Part print with two shaded views. Sizes in mm from the minimum x, y, z corner. Round coordinates to 2 decimals unless told otherwise and drop trailing zeros. Order: outer loops, then holes, each group sorted by start corner. A loop starts at its lowest first (then second) coordinate and runs counter-clockwise, first axis right, second up. Notation, with made-up numbers: M 52,-11 L 82,-11 A19 cw 82,22 Z; hole C 18,-36 d5. An arc over 180 degrees is marked long. Answer as a JSON object with one key per item and string values.
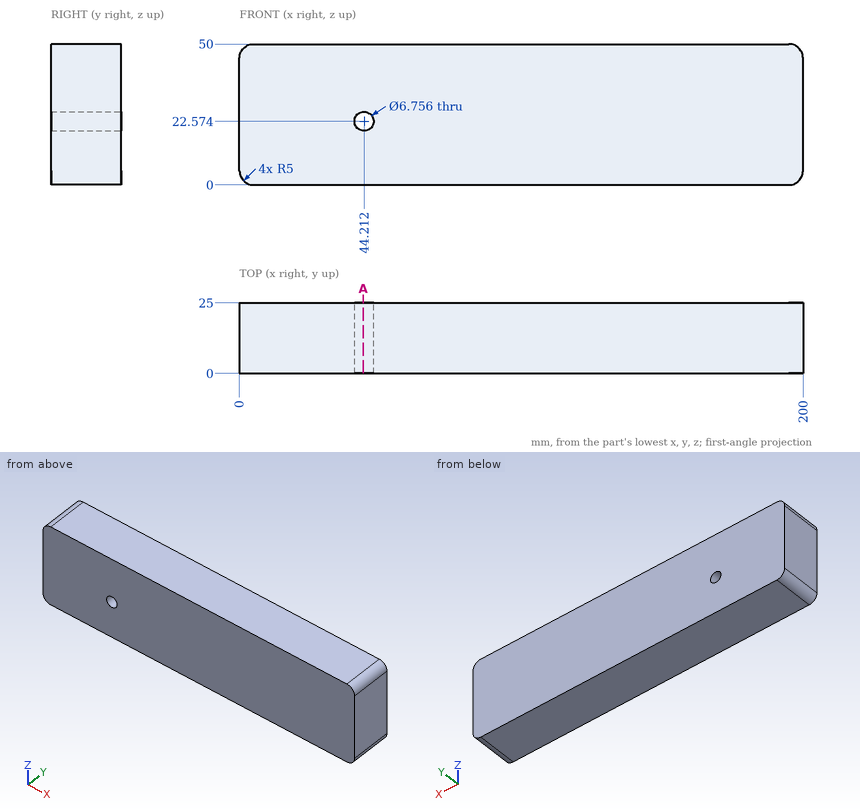
Item 1: Saw through at A-A on x = 44. List the corners of the cut face in (y, z) (1 decimal).
Worked answers:
{"outline": "M 0,0 L 25,0 L 25,19.2 L 0,19.2 Z; M 0,25.9 L 25,25.9 L 25,50 L 0,50 Z"}
Item 2: Wall check: line 1 along X through (y, z) = (16.25, 25.5) (1 decimal); line 2 along X through (y, z) = (7.25, 47.5). Give the ranges that are in metal, low to high. Write a range as [from, to].
Worked answers:
{"line 1": "x = [0, 42.5], [45.9, 200]", "line 2": "x = [0.67, 199.33]"}
Item 3: Drop flat-ended pins along their axis: pin 1 Ø5 at (x, z) = (120, 24.5) entering from -Y; pin 2 Ø4 at (x, z) = (44.21, 22.57) entering from -Y. Give the stop position or say it passes through.
Worked answers:
{"pin 1": "stops at y = 0", "pin 2": "passes through"}
